Work out the finished part from the listing and answer in its coordinate system (mm). Face numbers are marked on the shaded views. A direction names the side the tool comes from. Coordinates: 2 decimals unless noted, no trailing zeros. Order: outer loops, then holes, each group sorted by start corner. A loop starts at its lowest first (then second) coordinate and runs counter-clockwise, first axis right, second up.
1. A tool of negligible diameter and unlimited length cuts with its end or side. For the marked faces 4, 5, 6 and 7, from which of +Z, -Z, +X, -X, +Y, -Y can it reach the whole face along a straight path? Write none if from no direction.
2. The part is cut by section B-B, the plane y = 33. Give the vertices of the cut face in (x, z), then the cut area to 3 significant figures.
3. Flat-ended cylindrical pins translate along their axes: pin 1 Ø6 at (x, y) = (13, 52) entering from +Z; pin 2 Ø2 at (x, y) = (3, 51) entering from +Z; pin 3 Ø13 at (x, y) = (5.5, 17) entering from +Z. Find the tip coordinate at first contact, or state that the pin passes through.
4. Find the intervals of material crossed by probe 1 along X at (y, z) = (0.55, 32); probe 2 along Z at (x, y) = (11, 1.1); probe 3 along Y at (x, z) = (20.75, 18), in increasing order.
5. Determine the mould class of the marked faces 1, 2 and 3 for opening direction Y: +Y half, -Y half, draft (parallel to the pull), parting line (faces both ways), or undercut.
6. The part is cut by section C-C, the plane y = 40.5. Give the vertices of the cut face in (x, z).
7. The part is cut by section A-A, the plane x = 3.5. Count the separate pieces of the cut face and the enclosed holes in it, then the cut area to 3 significant figures.
```python
from build123d import *

# Parameters (mm, degrees)
F1_DEPTH  = 22
F2_R      = 5
F3_R      = 1
F4_R      = 1
F6_R      = 5
F7_DEPTH  = 47
F8_R      = 2.5
F9_DEPTH  = 50.001
F10_SIZE  = 1
F12_W     = 2
F12_H     = 14.2733568645
F13_DEPTH = 47
F16_DEPTH = 10
F17_R     = 0.5
F19_DEPTH = 22


with BuildPart() as f1:
    # F0 (on Right) → F1 (new body)
    with BuildSketch(Plane.YZ):
        with BuildLine():
            Line((3, 32), (3, 39))
            Line((3, 39), (0, 39))
            Line((0, 39), (0, 0))
            Line((0, 0), (57.4654344921, 0))
            ThreePointArc((57.4654344921, 0), (60.4687056177, 13.1164471126), (62.9455756953, 26.3424040508))
            Line((62.9455756953, 26.3424040508), (59, 27))
            Line((59, 27), (56, 9))
            ThreePointArc((56, 9), (42, 3), (28, 9))
            Line((28, 9), (25, 27))
            Line((25, 27), (7.8786796564, 27))
            Line((7.8786796564, 27), (5.7829372183, 27))
            Line((5.7829372183, 27), (3, 27))
            Line((3, 27), (3, 29.8521417825))
            Line((3, 29.8521417825), (3, 32))
        make_face()
        Polygon((19.3786796564, 1.5), (1.5, 1.5), (1.5, 19.3786796564), align=None, mode=Mode.SUBTRACT)
        Polygon((20, 3), (1.5, 21.5), (1.5, 25.5), (7.2573593129, 25.5), (29.7573593129, 3), align=None, mode=Mode.SUBTRACT)
        Polygon((25.9911590566, 8.8875205998), (9.3786796564, 25.5), (23.2224124899, 25.5), align=None, mode=Mode.SUBTRACT)
        Polygon((7.8786796564, 27), (3, 32), (3, 29.8521417825), (5.7829372183, 27), align=None)
    extrude(amount=F1_DEPTH)

    # F2
    f2_edges = [f1.edges().sort_by_distance(p)[0] for p in [
        (11, 57.465434, 0),
        (11, 56, 9),
        (11, 28, 9),
    ]]
    fillet(f2_edges, radius=F2_R)

    # F3
    f3_edges = [f1.edges().sort_by_distance(p)[0] for p in [
        (11, 59, 27),
        (11, 62.945576, 26.342404),
        (11, 3, 39),
        (11, 25, 27),
        (11, 23.222412, 25.5),
    ]]
    fillet(f3_edges, radius=F3_R)

    # F4
    f4_edges = [f1.edges().sort_by_distance(p)[0] for p in [
        (11, 1.5, 1.5),
        (11, 19.37868, 1.5),
        (11, 20, 3),
        (11, 1.5, 21.5),
        (11, 1.5, 19.37868),
        (11, 7.257359, 25.5),
        (11, 9.37868, 25.5),
        (11, 29.757359, 3),
        (11, 1.5, 25.5),
        (11, 25.991159, 8.887521),
    ]]
    fillet(f4_edges, radius=F4_R)

    # F6 (on offset) → F7 (cut, through all)
    with BuildSketch(Plane.XZ.offset(-50)):
        with Locations((11, 32)):
            Circle(F6_R)
    extrude(amount=F7_DEPTH, mode=Mode.SUBTRACT)

    # F8 (on offset) → F9 (cut, through all)
    with BuildSketch(Plane.XZ.offset(-50)):
        with Locations((11, 32)):
            Circle(F8_R)
    extrude(amount=F9_DEPTH, mode=Mode.SUBTRACT)

    # F10
    f10_edges = [f1.edges().sort_by_distance(p)[0] for p in [
        (8.5, 3, 32),
    ]]
    chamfer(f10_edges, length=F10_SIZE)

    # F12 (on offset) → F13 (cut)
    with BuildSketch(Plane.XY.offset(50)):
        with Locations((3.5, 49.1366784322)):
            Rectangle(F12_W, F12_H)
        with Locations((8.5, 49.1366784322)):
            Rectangle(F12_W, F12_H)
        with Locations((13.5, 49.1366784322)):
            Rectangle(F12_W, F12_H)
        with Locations((18.5, 49.1366784322)):
            Rectangle(F12_W, F12_H)
    extrude(amount=-F13_DEPTH, mode=Mode.SUBTRACT)

    # F15 (on offset) → F16 (cut, symmetric)
    with BuildSketch(Plane.YZ.offset(11)):
        Polygon((61.6930370138, 25.0304698651), (60.2329924048, 25.2738106333), (58.0149187036, 11.9653684263), (59.0013126275, 11.800969439), align=None)
    extrude(amount=F16_DEPTH, both=True, mode=Mode.SUBTRACT)

    # F17
    f17_edges = [f1.edges().sort_by_distance(p)[0] for p in [
        (11, 59.001313, 11.800969),
        (11, 60.232992, 25.273811),
        (11, 61.693037, 25.03047),
        (11, 58.014919, 11.965368),
    ]]
    fillet(f17_edges, radius=F17_R)

    # F18 (on face) → F19 (join, through all)
    with BuildSketch(Plane.YZ.offset(22)):
        with BuildLine():
            ThreePointArc((54.600010703, 7.6698580269), (42, 3), (29.399989297, 7.6698580269))
            Line((29.399989297, 7.6698580269), (28.7482646674, 6.9114024796))
            ThreePointArc((28.7482646674, 6.9114024796), (42, 2.000000095), (55.2517353326, 6.9114024796))
            ThreePointArc((55.2517353326, 6.9114024796), (56.568912669, 8.5171443059), (57.2597506946, 10.4757422152))
            Line((57.2597506946, 10.4757422152), (56.2733568645, 10.6401411869))
            ThreePointArc((56.2733568645, 10.6401411869), (55.6976585007, 9.0079762366), (54.600010703, 7.6698580269))
        make_face()
    extrude(amount=-F19_DEPTH)


solid = f1.part
```
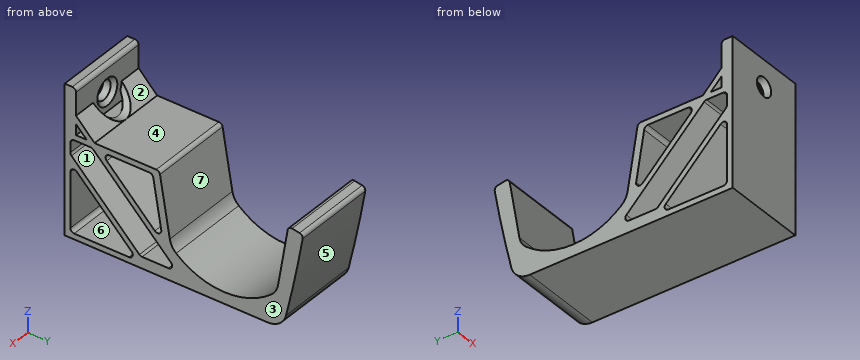
Geometry says:
1. face 4: +Z, +X, -X, +Y
1. face 5: -Z, +X, -X, +Y
1. face 6: +X, -X
1. face 7: +Z, +X, -X
2. outline: (0, 0) - (22, 0) - (22, 5.22) - (0, 5.22) - close
2. area: 115 mm2
3. pin 1: stops at z = 8.05
3. pin 2: stops at z = 5.79
3. pin 3: stops at z = 27
4. probe 1: x = 0 to 8.5, 13.5 to 22
4. probe 2: z = 0 to 29.5, 34.5 to 39
4. probe 3: y = 0 to 5, 14.76 to 16.88, 24.47 to 26.5, 57.5 to 59.02, 60.26 to 61.45
5. face 1: undercut
5. face 2: +Y half
5. face 3: draft
6. outline: (0, 0) - (22, 0) - (22, 3.06) - (0, 3.06) - close
7. separate pieces: 1
7. enclosed holes: 6
7. area: 486 mm2
